The listing builds one solid part. Answer for the finished solid, in the listing's coordinates (mm). Face numbers are marked on the shaded views. A direction names the side the tool comes from. Give positions to 0.01 mm unless a question says otherwise; leave off trailing zeros. Write each loop counter-clockwise with the first axis right and the second up, starting at its lowest first coordinate (ties: lowest second). Pieces come first, ordered by that corner, then holes. Notation, with made-up numbers: M 33,0 L 90,0 A20 ccw 90,11 Z; hole C 0.25,85 d1. An arc over 180 degrees is marked long. Answer as a JSON object with one key per item and string values.
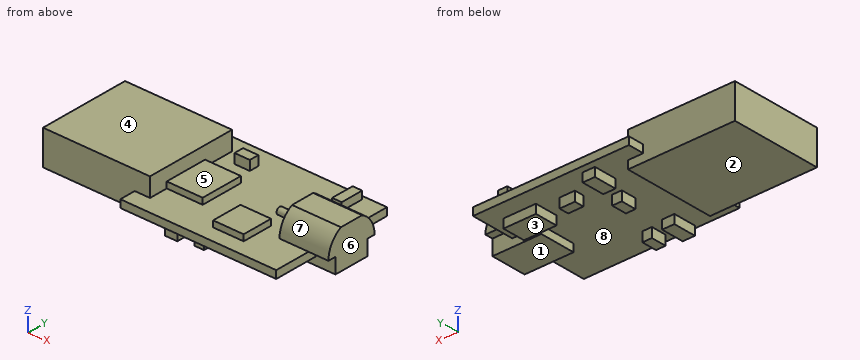
```python
from build123d import *

# Parameters (mm, degrees)
F0_W          = 20.4
F0_H          = 16.2
F1_DEPTH      = 1
F2_W          = 12
F2_H          = 4.5
F3_DEPTH      = 12
F3_DEPTH_BACK = 2
F4_W          = 4.7
F4_H          = 1
F5_DEPTH      = 2.6
F5_DEPTH_BACK = 3.8
F6_R          = 0.45
F7_DEPTH      = 3
F8_W          = 5.6
F8_H          = 5.6
F9_DEPTH      = 0.8
F10_W         = 4
F10_H         = 4
F11_DEPTH     = 0.8
F12_W         = 2
F12_H         = 1.25
F13_DEPTH     = 1.25
F14_W         = 1.25
F14_H         = 3
F15_DEPTH     = 1
F16_W         = 2
F16_H         = 1.25
F16_W_2       = 1.25
F16_H_2       = 2
F17_DEPTH     = 1.25
F18_W         = 1.6
F18_H         = 3
F19_DEPTH     = 1.15
F20_W         = 4.25
F20_H         = 3
F21_DEPTH     = 1.15


with BuildPart() as f1:
    # F0 (on Top) → F1 (new body)
    with BuildSketch(Plane.XY):
        Rectangle(F0_W, F0_H)
    extrude(amount=-F1_DEPTH)

    # F2 (on face) → F3 (join, two sides)
    with BuildSketch(Plane(origin=(-10.2, 0, 0), x_dir=(0, -1, 0), z_dir=(-1, 0, 0))) as f3_sk:
        with Locations((0, 0.2)):
            Rectangle(F2_W, F2_H)
    extrude(amount=F3_DEPTH)
    extrude(f3_sk.sketch, amount=-F3_DEPTH_BACK)

    # F4 (on face) → F5 (join, two sides)
    with BuildSketch(Plane.YZ.offset(10.2)) as f5_sk:
        with Locations((0, -1.5)):
            Rectangle(F4_W, F4_H)
        with Locations((0, -0.5)):
            Rectangle(F4_W, F4_H)
        with BuildLine():
            Line((-3.375, 0), (-2.35, 0))
            Line((-2.35, 0), (2.35, 0))
            Line((2.35, 0), (3.375, 0))
            ThreePointArc((3.375, 0), (2.8817469144, 1.7567469144), (1.5461646096, 3))
            Line((1.5461646096, 3), (-1.5461646096, 3))
            ThreePointArc((-1.5461646096, 3), (-2.8817469144, 1.7567469144), (-3.375, 0))
        make_face()
    extrude(amount=F5_DEPTH)
    extrude(f5_sk.sketch, amount=-F5_DEPTH_BACK)

    # F6 (on face) → F7 (join)
    with BuildSketch(Plane(origin=(6.4, 0, 0), x_dir=(0, -1, 0), z_dir=(-1, 0, 0))):
        with Locations((0, 0.5)):
            Circle(F6_R)
    extrude(amount=F7_DEPTH)

    # F8 (on face) → F9 (join)
    with BuildSketch(Plane.XY):
        with Locations((-6.3, -0.75)):
            Rectangle(F8_W, F8_H)
    extrude(amount=F9_DEPTH)

    # F10 (on face) → F11 (join)
    with BuildSketch(Plane.XY):
        with Locations((2.15, -4.1)):
            Rectangle(F10_W, F10_H)
    extrude(amount=F11_DEPTH)

    # F12 (on face) → F13 (join)
    with BuildSketch(Plane.XY):
        with Locations((-5.4, 4.975)):
            Rectangle(F12_W, F12_H)
    extrude(amount=F13_DEPTH)

    # F14 (on face) → F15 (join)
    with BuildSketch(Plane.XY):
        with Locations((6.775, 6.1)):
            Rectangle(F14_W, F14_H)
    extrude(amount=F15_DEPTH)

    # F16 (on face) → F17 (join)
    with BuildSketch(Plane(origin=(0, 0, -1), x_dir=(1, 0, 0), z_dir=(0, 0, -1))):
        with Locations((0.55, -4.475)):
            Rectangle(F16_W, F16_H)
        with Locations((-3.275, -1.1)):
            Rectangle(F16_W_2, F16_H_2)
        with Locations((-0.775, 6.1)):
            Rectangle(F16_W_2, F16_H_2)
    extrude(amount=F17_DEPTH)

    # F18 (on face) → F19 (join)
    with BuildSketch(Plane(origin=(0, 0, -1), x_dir=(1, 0, 0), z_dir=(0, 0, -1))):
        with Locations((-4.15, -5.7)):
            Rectangle(F18_W, F18_H)
        with Locations((-3.9, 6.2)):
            Rectangle(F18_W, F18_H)
    extrude(amount=F19_DEPTH)

    # F20 (on face) → F21 (join)
    with BuildSketch(Plane(origin=(0, 0, -1), x_dir=(1, 0, 0), z_dir=(0, 0, -1))):
        with Locations((6.175, -4.27)):
            Rectangle(F20_W, F20_H)
    extrude(amount=F21_DEPTH)


solid = f1.part
```
1. Flat-ended cylindrical pins translate along their axes: pin 1 (8 mm diameter, centred on x = 7.5, y = 1.5, fed in from -Z); pin 2 (1.5 mm diameter, centred on x = 3, y = -1, fed in from -Z); pin 3 (2 mm diameter, centred on y = 5.5, z = -1, fed in from +X). Find the tip coordinate at first contact, or state that the pin passes through.
Verdict:
{"pin 1": "stops at z = -2.15", "pin 2": "stops at z = -1", "pin 3": "stops at x = 10.2"}
2. A cutting plane is placed at B-B, the plane y = -5.5. Give the vertices of the cut face in (x, z), plus the area to 3 significant figures.
Verdict:
{"outline": "M -22.2,-2.05 L -8.2,-2.05 L -8.2,-1 L -4.7,-1 L -4.7,-2.15 L -3.1,-2.15 L -3.1,-1 L -1.4,-1 L -1.4,-2.25 L -0.15,-2.25 L -0.15,-1 L 10.2,-1 L 10.2,0 L 4.15,0 L 4.15,0.8 L 0.15,0.8 L 0.15,0 L -8.2,0 L -8.2,2.45 L -22.2,2.45 Z", "area": "88.0 mm2"}
3. A cutting plane is placed at C-C, the plane x = -13. Give the vertices of the cut face in (y, z).
Verdict:
{"outline": "M -6,-2.05 L 6,-2.05 L 6,2.45 L -6,2.45 Z"}
4. The mould has two halves that part along X. Classify the marked faces 6, 7 and 8: released by +X, released by -X, zero draft, split by the parting line, or undercut.
Verdict:
{"face 6": "released by +X", "face 7": "zero draft", "face 8": "undercut"}
5. For the marked faces 1, 2, 3, 4 and 5, determine the directions among +Z, -Z, +X, -X, +Y, -Y from which every point of the face is accessible in a straight line to the end or side of a thin tool.
Verdict:
{"face 1": "-Z, +X, -Y", "face 2": "-Z, -X, +Y, -Y", "face 3": "-Z, +X, +Y, -Y", "face 4": "+Z, -X, +Y, -Y", "face 5": "+Z, -Y"}
6. Consider line 1 along X through (y, z) = (1, -1.55); line 2 along X through (y, z) = (-1, -1.65); line 3 along X through (y, z) = (-1.5, 0.55). Determine where each line is inside the solid, lowest interval first.
Verdict:
{"line 1": "x = -22.2 to -8.2, -3.9 to -2.65, 6.4 to 12.8", "line 2": "x = -22.2 to -8.2, 6.4 to 12.8", "line 3": "x = -22.2 to -3.5, 6.4 to 12.8"}
7. A cutting plane is placed at A-A, the plane z = 2. Give the vertices of the cut face in (x, y).
Verdict:
{"outline": "M -22.2,-6 L -8.2,-6 L -8.2,6 L -22.2,6 Z; M 6.4,-2.72 L 12.8,-2.72 L 12.8,2.72 L 6.4,2.72 Z"}
